The model under review builds one solid part; all positions refer to its coordinate system, in mm. A direction names the side the tool comes from. Round coordinates to 2 decimals unless told otherwise and drop trailing zeros. Order: outer loops, then holes, each group sorted by start corner. A loop starts at its lowest first (then second) coordinate and runs counter-clockwise, first axis right, second up. Notation, with made-up numbers: M 13,-22.5 L 53,-22.5 A21 cw 53,-18.5 Z; hole C 39.25,25.5 d6. An arc over 180 degrees is marked long. Answer as a JSON object with one key per item and string values. Group by question number.
1) Consider section A-A, the plane z = -73.66. Write out the cut boundary in (x, y), then the cut area to 3 significant figures.
2) For faces 4 (the flat face through (30, -9.136, -102)), 5 (the flat face through (12, -7.927, -2)), 6 (the cylindrical face through (28.17, -10.79, -56.03)), 7 (the cylindrical face through (0.738, -0.699, -51.412)), list the 3-axis set-ups (+Z, -Z, +X, -X, +Y, -Y) from which the entire face can be reached by the end or side of a thin tool; tool diameter is ignored.
3) Consider section C-C, the plane z = -45.5. Write out the cut boundary in (x, y), then the cut area to 3 significant figures.
4) Consider section B-B, the plane x = 30.48. Write out the cut boundary in (y, z).
5) Consider section D-D, the plane x = 18.5. Write out the cut boundary in (y, z), then the cut area to 3 significant figures.
6) To check wall thickness, follow line 1 (Z direction, x = 30.48, y = -10.8); line 2 (Y direction, x = 28.5, z = -100); line 3 (Z direction, x = 17, y = -8.75). State the ranges of each line that lie inside material, in increasing order.
7) Insertion check: pin 1 Ø1.9 at (y, z) = (-8.5, -103) entering from +X; pin 2 Ø0.5 at (y, z) = (-9, -2.5) entering from -X; pin 3 Ø1 at (x, z) = (48.5, -46.5) entering from -Y. Each pin has a flat end and moves straight along its axis. Give the tip position at first contact, or say it passes through.
8) The part is to be moulded in two halves that separate along Z. For faces 1 (the cylindrical face through (30.124, -0.699, -103.402)), 2 (the flat face through (12, -9.467, -2)), 3 (the cylindrical face through (34.576, -10.79, -67.235)), say which applies: +Z half, -Z half, draft (parallel to the pull), parting line (faces both ways), or undercut.
```python
from build123d import *

# Parameters (mm, degrees)
F0_W      = 60.96
F0_H      = 104.14
F1_DEPTH  = 10.414
F2_R      = 5.08
F3_W      = 53.34
F3_H      = 38.1
F3_R      = 17.78
F3_R_2    = 7.62
F4_DEPTH  = 0.762
F5_R      = 2.4528409794
F7_R      = 0.9755927776
F7_W      = 10.8667761087
F7_H      = 1.5401728451
F8_DEPTH  = 4.318
F9_W      = 29.0065901354
F9_H      = 1.7113029025
F10_DEPTH = 4.064


with BuildPart() as f1:
    # F0 (on Front) → F1 (new body)
    with BuildSketch(Plane.XZ):
        with Locations((30.48, -52.07)):
            Rectangle(F0_W, F0_H)
    extrude(amount=F1_DEPTH)

    # F2
    f2_edges = [f1.edges().sort_by_distance(p)[0] for p in [
        (60.96, -5.207, 0),
        (0, -5.207, 0),
        (0, -5.207, -104.14),
        (60.96, -5.207, -104.14),
    ]]
    fillet(f2_edges, radius=F2_R)

    # F3 (on face) → F4 (join)
    with BuildSketch(Plane.XZ.offset(10.414)):
        with Locations((30.48, -25.4)):
            Rectangle(F3_W, F3_H)
        with Locations((30.48, -73.66)):
            Circle(F3_R)
        with Locations((30.48, -73.66)):
            Circle(F3_R_2, mode=Mode.SUBTRACT)
    extrude(amount=F4_DEPTH)

    # F5
    f5_edges = [f1.edges().sort_by_distance(p)[0] for p in [
        (1.487898, 0, -1.487898),
    ]]
    fillet(f5_edges, radius=F5_R)

    # F7 (on face) → F8 (cut)
    with BuildSketch(Plane.XY):
        with Locations((56.6684938967, -6.9853682071)):
            Circle(F7_R)
        with Locations((11.6184335202, -8.6966715753)):
            Rectangle(F7_W, F7_H)
    extrude(amount=-F8_DEPTH, mode=Mode.SUBTRACT)

    # F9 (on face) → F10 (cut)
    with BuildSketch(Plane(origin=(0, 0, -104.14), x_dir=(1, 0, 0), z_dir=(0, 0, -1))):
        with Locations((30.1111503504, 8.2802635152)):
            Rectangle(F9_W, F9_H)
    extrude(amount=-F10_DEPTH, mode=Mode.SUBTRACT)


solid = f1.part
```
Results list:
{
 "1": {"outline": "M 0,-10.41 L 12.7,-10.41 L 12.7,-11.18 L 22.86,-11.18 L 22.86,-10.41 L 38.1,-10.41 L 38.1,-11.18 L 48.26,-11.18 L 48.26,-10.41 L 60.96,-10.41 L 60.96,-2.45 A2.45 ccw 58.51,0 L 2.45,0 A2.45 ccw 0,-2.45 Z", "area": "648 mm^2"},
 "2": {"face 4": "-Z", "face 5": "+Z", "face 6": "-Y", "face 7": "+Z, -Z, -X, +Y"},
 "3": {"outline": "M 0,-10.41 L 60.96,-10.41 L 60.96,-2.45 A2.45 ccw 58.51,0 L 2.45,0 A2.45 ccw 0,-2.45 Z", "area": "632 mm^2"},
 "4": {"outline": "M -11.18,-91.44 L -10.41,-91.44 L -10.41,-104.14 L -9.14,-104.14 L -9.14,-100.08 L -7.42,-100.08 L -7.42,-104.14 L -2.45,-104.14 A2.45 ccw 0,-101.69 L 0,-2.45 A2.45 ccw -2.45,0 L -10.41,0 L -10.41,-6.35 L -11.18,-6.35 L -11.18,-44.45 L -10.41,-44.45 L -10.41,-55.88 L -11.18,-55.88 L -11.18,-66.04 L -10.41,-66.04 L -10.41,-81.28 L -11.18,-81.28 Z"},
 "5": {"outline": "M -11.18,-86.8 L -10.41,-86.8 L -10.41,-104.14 L -9.14,-104.14 L -9.14,-100.08 L -7.42,-100.08 L -7.42,-104.14 L -2.45,-104.14 A2.45 ccw 0,-101.69 L 0,-2.45 A2.45 ccw -2.45,0 L -10.41,0 L -10.41,-6.35 L -11.18,-6.35 L -11.18,-44.45 L -10.41,-44.45 L -10.41,-60.52 L -11.18,-60.52 Z", "area": "1,120 mm^2"},
 "6": {"line 1": "-91.44 to -81.28, -66.04 to -55.88, -44.45 to -6.35", "line 2": "-10.41 to 0", "line 3": "-100.08 to -4.32"},
 "7": {"pin 1": "x = 59.99", "pin 2": "x = 0.57", "pin 3": "y = -10.41"},
 "8": {"face 1": "-Z half", "face 2": "draft", "face 3": "undercut"}
}
